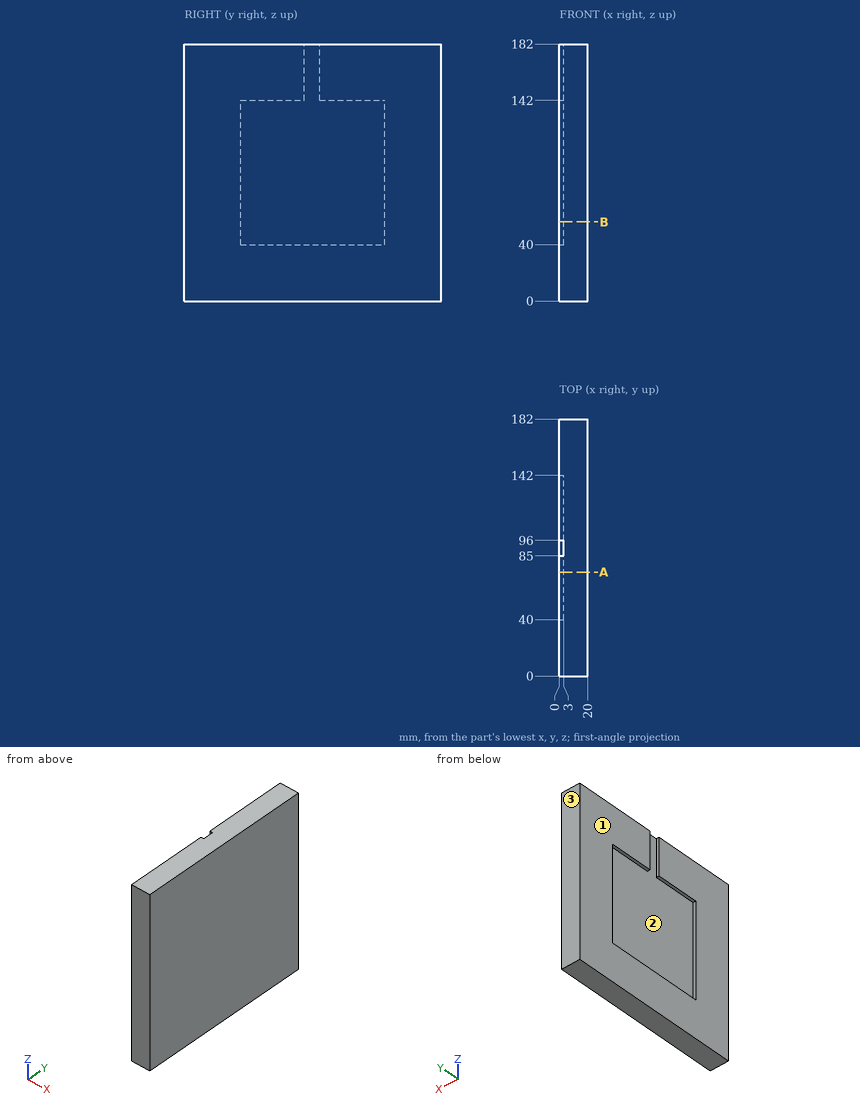
Verification items for this drawing (mm, ordinates from the low corner). Coordinates: 2 decimals unless noted, no trailing zeros. Order: outer loops, then holes, each group sorted by start corner. A loop starts at its lowest first (then second) coordinate and runs counter-clockwise, first axis right, second up. Notation, with made-up numbers: (82.5, 58.5) - (133.5, 58.5) arc R25 ccw to (133.5, 77.5) - close; hole circle Ø5 at (19, 10.25). An arc over 180 degrees is marked (long way). Use one line per item in the form item = value.
1. Scan lines: line 1 (Y direction, x = 1.25, z = 132.5); line 2 (X direction, y = 88.5, z = 76.5). Record each from-to range of solid material in increasing order.
Here are the results:
line_1 = 0 to 40, 142 to 182
line_2 = 3 to 20
2. Draft check along Y on the marked faces 1, 2 and 3. Enter one of: pulls with the +Y half, pulls with the -Y half, needs draft (parallel to the pull), parting line crosses it, or undercut.
Here are the results:
face_1 = needs draft
face_2 = undercut
face_3 = pulls with the +Y half
3. Gauge pin test, flat ends, axial feed: pin 1 (5 mm diameter, centred on y = 132, z = 67.5, fed in from -X); pin 2 (1.5 mm diameter, centred on x = 1, y = 92.5, fed in from +Z). Record the tip position at first contact, or that the pin passes through.
Here are the results:
pin_1 = 3
pin_2 = 40
4. Section check A-A (y = 73.5). Record the boundary of the cut face in (x, z), then the cut area to 3 significant figures.
Here are the results:
outline = (0, 0) - (20, 0) - (20, 182) - (0, 182) - (0, 142) - (3, 142) - (3, 40) - (0, 40) - close
area = 3,330 mm²
